Read the model definition and answer for the solid it produces. Units are mm, in the model's axes. Face numbers are marked on the shaded views. Coordinates: 2 decimals unless noted, no trailing zeros. Order: outer loops, then holes, each group sorted by start corner. A loop starts at its lowest first (then second) coordinate and runs counter-clockwise, first axis right, second up.
```python
from build123d import *

# Parameters (mm, degrees)
F0_W     = 18
F0_H     = 40
F0_W_2   = 11
F0_W_3   = 22
F1_DEPTH = 4.5
F2_W     = 11
F2_H     = 40
F3_DEPTH = 2
F5_DEPTH = 70
F6_R     = 2.49999


# Not quite as in the source:
# - a fillet or chamfer is up to 0.001 mm smaller than in the source, because OpenCascade refuses the exact size


with BuildPart() as f1:
    # F0 (on Front) → F1 (new body)
    with BuildSketch(Plane.XZ):
        with Locations((-31, 0)):
            Rectangle(F0_W, F0_H)
        with Locations((-16.5, 0)):
            Rectangle(F0_W_2, F0_H)
        Rectangle(F0_W_3, F0_H)
        with Locations((16.5, 0)):
            Rectangle(F0_W_2, F0_H)
        with Locations((31, 0)):
            Rectangle(F0_W, F0_H)
    extrude(amount=-F1_DEPTH)

    # F2 (on Front) → F3 (cut)
    with BuildSketch(Plane.XZ):
        with Locations((-16.5, 0)):
            Rectangle(F2_W, F2_H)
        with Locations((16.5, 0)):
            Rectangle(F2_W, F2_H)
    extrude(amount=-F3_DEPTH, mode=Mode.SUBTRACT)

    # F4 (on face) → F5 (cut)
    with BuildSketch(Plane(origin=(-40, 0, 0), x_dir=(0, -1, 0), z_dir=(-1, 0, 0))):
        Polygon((0, -2.5), (0, 0), (0, 2.5), (-1.5, 4), (-1.5, 0), (-1.5, -4), align=None)
    extrude(amount=-F5_DEPTH, mode=Mode.SUBTRACT)

    # F6 (radius 2.5 in the source; OpenCascade refuses exactly that, so slightly less here)
    f6_edges = [f1.edges().sort_by_distance(p)[0] for p in [
        (-16.5, 2, 20),
        (16.5, 2, 20),
        (16.5, 2, -20),
        (-16.5, 2, -20),
        (-40, 2.25, 20),
        (-40, 2.25, -20),
        (40, 2.25, -20),
        (40, 2.25, 20),
    ]]
    fillet(f6_edges, radius=F6_R)


solid = f1.part
```
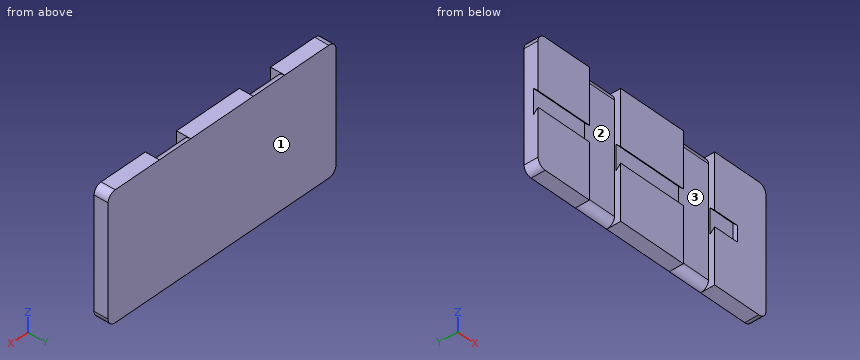
1) Straight lines are drawn through the part: line 1 (X direction, y = 0.45, z = 14); line 2 (Y direction, x = 27, z = 0); line 3 (X direction, y = 1.1, z = 1). For each, find the intervals that lie inside material, in ascending order.
A:
line 1: x = -40 to -22, -11 to 11, 22 to 40
line 2: y = 1.5 to 4.5
line 3: x = 30 to 40
2) Determine the mould class of the marked faces 1, 2 and 3 for opening direction X: pulls with the +X half, pulls with the -X half, needs draft (parallel to the pull), parting line crosses it, or undercut.
A:
face 1: needs draft
face 2: undercut
face 3: undercut
3) A cutting plane is placed at A-A, the plane x = 9. Determine the outline of the cut face in (y, z), and give its area (3 significant figures).
A:
outline: (0, -20) - (4.5, -20) - (4.5, 20) - (0, 20) - (0, 2.5) - (1.5, 4) - (1.5, -4) - (0, -2.5) - close
area: 170 mm2
4) A cutting plane is placed at B-B, the plane z = -7. Determine the outline of the cut face in (x, y).
A:
outline: (-40, 0) - (-22, 0) - (-22, 2) - (-11, 2) - (-11, 0) - (11, 0) - (11, 2) - (22, 2) - (22, 0) - (40, 0) - (40, 4.5) - (-40, 4.5) - close
5) A flat-ended cylindrical pin translates along its axis: pin 1 Ø5 at (x, z) = (19, -9) entering from -Y. Find the tip coordinate at first contact, or state that the pin passes through.
A:
pin 1: stops at y = 2
